Job drawing, mm, ordinate dimensions from the low corner. One solid piece. A direction names the side the tool comes from. Give positions to 0.01 mm unless a question says otherwise; leave off trailing zeros. Write each loop counter-clockwise with the first axis right and the second up, starting at its lowest first coordinate (ties: lowest second). Pieces come first, ordered by that corner, then holes. Notation, with made-up numbers: (-13.5, 47.25) -> (31.5, 47.25) arc R24 ccw to (31.5, 64.25) -> close; hole circle Ø5 at (19, -14.5). An arc over 180 degrees is marked (long way). One line per question, with ' | ' between items. Start each with the question number.
(1) Band-saw the part on B-B, the plane y = 6.75. Give the cut face in (x, z).
(2) Pull direction Z, two halves, no side cores. Call the marked faces 3, 4 and 5: released by +Z, released by -Z, zero draft, split by the parting line, or undercut.
(3) Band-saw the part on A-A, the plane x = 5. Give the cut face in (y, z), and give its area (3 significant figures).
(4) Band-saw the part on D-D, the plane x = 31. Give the cut face in (y, z).
(5) Tool access for the marked faces 1 and 2: list every direction of +Z, -Z, +X, -X, +Y, -Y with a clear straight run to the whole face (end or side of a thin tool).
(6) Band-saw the part on C-C, the plane y = 11.5. Give the cut face in (x, z).
(7) Pin check, flat tip, straight feed: P1, Ø1, axis at x = 28, z = 11, coming from the -Y side. Stop position of the tip, or through.
(8) Drill centre lines: probe 1 along Z at (x, y) = (12.5, 18.75); probe 2 along Y at (x, z) = (19, 39.5); probe 3 along Y at (x, z) = (5, 42.05). Where is each one in solid material? Low to high. Write a range as from..to.
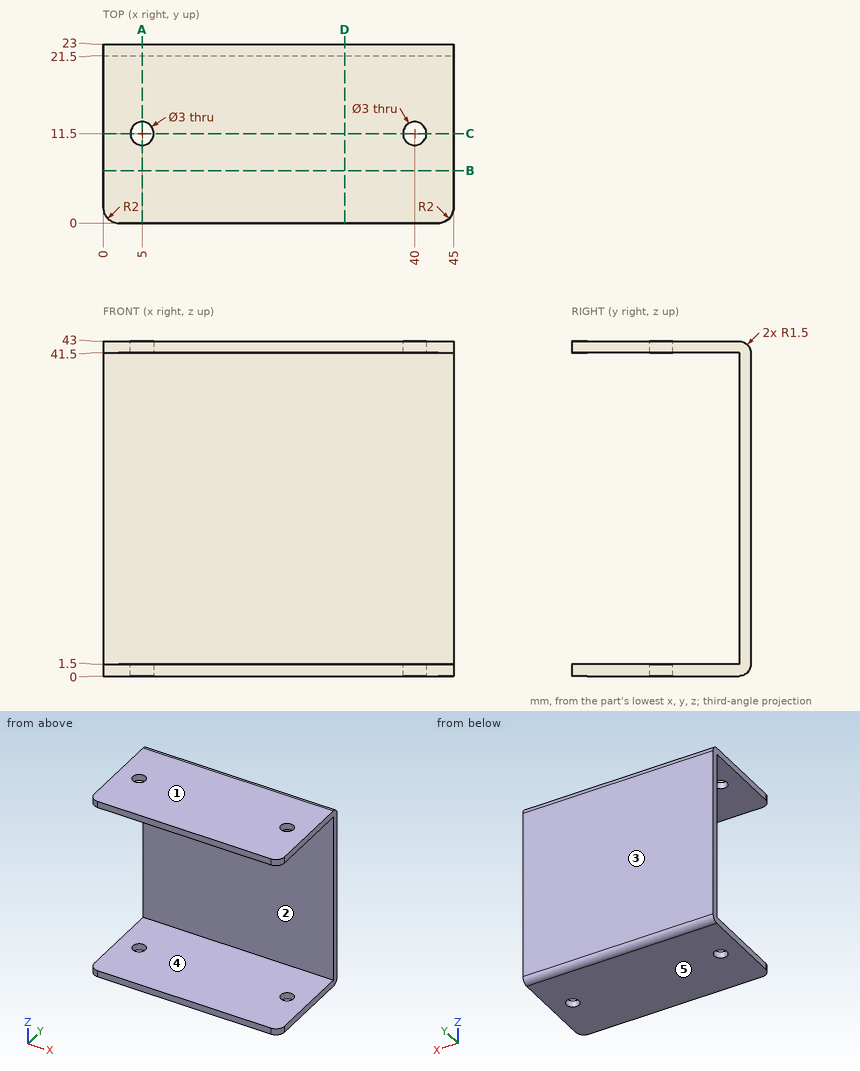
Results:
1) outline: (0, 0) -> (45, 0) -> (45, 1.5) -> (0, 1.5) -> close; (0, 41.5) -> (45, 41.5) -> (45, 43) -> (0, 43) -> close
2) face 3: zero draft | face 4: undercut | face 5: released by -Z
3) outline: (0, 0) -> (10, 0) -> (10, 1.5) -> (0, 1.5) -> close; (0, 41.5) -> (10, 41.5) -> (10, 43) -> (0, 43) -> close; (13, 0) -> (21.5, 0) arc R1.5 ccw to (23, 1.5) -> (23, 41.5) arc R1.5 ccw to (21.5, 43) -> (13, 43) -> (13, 41.5) -> (21.5, 41.5) -> (21.5, 1.5) -> (13, 1.5) -> close | area: 119 mm²
4) outline: (0, 0) -> (21.5, 0) arc R1.5 ccw to (23, 1.5) -> (23, 41.5) arc R1.5 ccw to (21.5, 43) -> (0, 43) -> (0, 41.5) -> (21.5, 41.5) -> (21.5, 1.5) -> (0, 1.5) -> close
5) face 1: +Z, +X, -X, +Y, -Y | face 2: +X, -X, -Y
6) outline: (0, 0) -> (3.5, 0) -> (3.5, 1.5) -> (0, 1.5) -> close; (0, 41.5) -> (3.5, 41.5) -> (3.5, 43) -> (0, 43) -> close; (6.5, 0) -> (38.5, 0) -> (38.5, 1.5) -> (6.5, 1.5) -> close; (6.5, 41.5) -> (38.5, 41.5) -> (38.5, 43) -> (6.5, 43) -> close; (41.5, 0) -> (45, 0) -> (45, 1.5) -> (41.5, 1.5) -> close; (41.5, 41.5) -> (45, 41.5) -> (45, 43) -> (41.5, 43) -> close
7) P1: stops at y = 21.5
8) probe 1: z = 0..1.5, 41.5..43 | probe 2: y = 21.5..23 | probe 3: y = 0..10, 13..22.9
